Check sheet for the modelled part. Datum: model origin and axes. Units: mm. A direction names the side the tool comes from. Round coordinates to 2 decimals unless told otherwise and drop trailing zeros. Loops run counter-clockwise (first coordinate to the right, second up) from the corner with the lowest first, then second, coordinate; pieces in that order, holes last. Notation, with made-up numbers: (-8, -5) - (23, -5) arc R32 ccw to (23, 26) - close; hole circle Ø3 at (7.25, 71.25). An arc over 180 degrees is marked (long way). Put each result on its own line as item: value. Start each with the question number.
Item 1: Section check C-C, the plane y = 1.25. Give the number of separate pieces and of enclosed holes in the cut face, and give its area (3 significant figures).
Item 2: Tool access check on faces 5 (the flat face through (-23.768, 6, -4)), 6 (the flat face through (-7, 3, 15.211)), 7 (the cylindrical face through (-31.67, 3.11, 14.64)), 8 (the flat face through (3, 2, -2.789)), 9 (the flat face through (7.832, 6, -16)). Record the directions out of +Z, -Z, +X, -X, +Y, -Y that give a thin tool (end or side, any length) a straight path to the whole face; none if there is none.
Item 3: Section check A-A, the plane z = 3.5. Record the cut outline in (x, y), and give its area (3 significant figures).
Item 4: Gauge pin test, flat ends, axial feed: pin 1 Ø0.5 at (x, y) = (0, 2.5) entering from -Z; pin 2 Ø2 at (y, z) = (2.5, -8) entering from -X; pin 3 Ø2 at (y, z) = (3.5, 1) entering from +X; pin 4 Ø3 at (x, y) = (-4.5, 7) entering from -Z. Record the tip position at first contact, or that the pin passes through.
Item 5: Section check B-B, the plane x = 13. Record the cut outline in (y, z), and give its area (3 significant figures).
Item 6: Draft check along Z on faces 1 (the cylindrical face through (17.13, 3.11, 14.64)), 2 (the flat face through (-18, 2, -16.789)), 3 (the flat face through (-32.268, 3, -4)), 4 (the flat face through (-14, 2, -16.789)). Enter one of: pulls with the +Z half, pulls with the -Z half, needs draft (parallel to the pull), parting line crosses it, or undercut.
Item 7: Material ranges on line 1 along Z through (x, y) = (0, 6); line 2 along X through (y, z) = (5, -6.5); line 3 along Y through (x, z) = (2.5, -29), recorded low to high.
from build123d import *
from build123d.topology import SkipClean

# Parameters (mm, degrees)
SKETCH_1_W          = 54
SKETCH_1_H          = 54
EXTRUDE_2_DEPTH     = 2.2
SKETCH_7_W          = 50
SKETCH_7_H          = 50
EXTRUDE_3_DEPTH     = 1.8
EXTRUDE_5_DEPTH     = 4
SKETCH_9_8_W        = 1.5
SKETCH_9_8_H        = 7
SKETCH_9_8_H_2      = 14
CUT_EXTRUDE_2_DEPTH = 10
FILLET_1_R          = 2
SKETCH_15_W         = 0.001
SKETCH_15_H         = 1.8
REVOLVE_8_ANGLE     = 332


with BuildPart() as part:
    # 草图1 → 凸台-拉伸2 (new body)
    with BuildSketch(Plane(origin=(0, 0, 0), x_dir=(1, 0, 0), z_dir=(0, 1, 0))):
        with Locations((-7.2681601, 9.789048154)):
            Rectangle(SKETCH_1_W, SKETCH_1_H)
    extrude(amount=EXTRUDE_2_DEPTH)

    # 草图7 → 凸台-拉伸3 (add)
    with BuildSketch(Plane(origin=(0, 2.2, 0), x_dir=(1, 0, 0), z_dir=(0, 1, 0))):
        with Locations((-7.2681601, 9.789048154)):
            Rectangle(SKETCH_7_W, SKETCH_7_H)
    extrude(amount=EXTRUDE_3_DEPTH)

    # 草图9 → 凸台-拉伸5 (add)
    with BuildSketch(Plane(origin=(0, 4, 0), x_dir=(1, 0, 0), z_dir=(0, 1, 0))):
        with BuildLine():
            Line((-22.7681601, -1.710951846), (8.2318399, -1.710951846))
            ThreePointArc((8.2318399, -1.710951846), (8.938946681, -1.418058627), (9.2318399, -0.710951846))
            Line((9.2318399, -0.710951846), (9.2318399, 7.789048154))
            Line((9.2318399, 7.789048154), (7.8318399, 7.789048154))
            Line((7.8318399, 7.789048154), (7.8318399, -0.310951846))
            Line((7.8318399, -0.310951846), (-22.3681601, -0.310951846))
            Line((-22.3681601, -0.310951846), (-22.3681601, 7.789048154))
            Line((-22.3681601, 7.789048154), (-23.7681601, 7.789048154))
            Line((-23.7681601, 7.789048154), (-23.7681601, -0.710951846))
            ThreePointArc((-23.7681601, -0.710951846), (-23.475266881, -1.418058627), (-22.7681601, -1.710951846))
        make_face()
        with BuildLine():
            Line((-22.7681601, 21.289048154), (8.2318399, 21.289048154))
            ThreePointArc((8.2318399, 21.289048154), (8.938946681, 20.996154935), (9.2318399, 20.289048154))
            Line((9.2318399, 20.289048154), (9.2318399, 11.789048154))
            Line((9.2318399, 11.789048154), (7.8318399, 11.789048154))
            Line((7.8318399, 11.789048154), (7.8318399, 19.889048154))
            Line((7.8318399, 19.889048154), (-22.3681601, 19.889048154))
            Line((-22.3681601, 19.889048154), (-22.3681601, 11.789048154))
            Line((-22.3681601, 11.789048154), (-23.7681601, 11.789048154))
            Line((-23.7681601, 11.789048154), (-23.7681601, 20.289048154))
            ThreePointArc((-23.7681601, 20.289048154), (-23.475266881, 20.996154935), (-22.7681601, 21.289048154))
        make_face()
    extrude(amount=EXTRUDE_5_DEPTH)

    # 草图9<8> → 切除-拉伸2 (cut)
    with BuildSketch(Plane(origin=(0, 4, 0), x_dir=(1, 0, 0), z_dir=(0, 1, 0))):
        with Locations((-10.7681601, 13.289048154)):
            Rectangle(SKETCH_9_8_W, SKETCH_9_8_H)
        with Locations((-10.7681601, 6.289048154)):
            Rectangle(SKETCH_9_8_W, SKETCH_9_8_H)
        with Locations((-7.2681601, 9.789048154)):
            Rectangle(SKETCH_9_8_W, SKETCH_9_8_H_2)
        with Locations((-14.2681601, 9.789048154)):
            Rectangle(SKETCH_9_8_W, SKETCH_9_8_H_2)
        with Locations((-17.7681601, 9.789048154)):
            Rectangle(SKETCH_9_8_W, SKETCH_9_8_H_2)
        with Locations((-3.7681601, 9.789048154)):
            Rectangle(SKETCH_9_8_W, SKETCH_9_8_H_2)
        with Locations((-0.2681601, 9.789048154)):
            Rectangle(SKETCH_9_8_W, SKETCH_9_8_H_2)
        with Locations((3.2318399, 9.789048154)):
            Rectangle(SKETCH_9_8_W, SKETCH_9_8_H_2)
    extrude(amount=-CUT_EXTRUDE_2_DEPTH, mode=Mode.SUBTRACT)

    # 圆角1
    fillet_1_edges = [part.edges().sort_by_distance(p)[0] for p in [
        (17.7318399, 3.1, 15.210951846),
        (17.7318399, 3.1, -34.789048154),
        (-32.2681601, 3.1, -34.789048154),
        (-32.2681601, 3.1, 15.210951846),
        (-34.2681601, 1.1, -36.789048154),
        (19.7318399, 1.1, -36.789048154),
        (19.7318399, 1.1, 17.210951846),
        (-34.2681601, 1.1, 17.210951846),
    ]]
    fillet(fillet_1_edges, radius=FILLET_1_R)

    # 草图12 → 旋转-薄壁5 (revolve)
    with BuildSketch(Plane.XY.offset(15.210951846)):
        with BuildLine():
            ThreePointArc((-7.2681601, 2.35), (-6.5181601, 3.1), (-7.2681601, 3.85))
            Line((-7.2681601, 3.85), (-7.2681601, 3.851))
            ThreePointArc((-7.2681601, 3.851), (-6.5171601, 3.1), (-7.2681601, 2.349))
            Line((-7.2681601, 2.349), (-7.2681601, 2.35))
        make_face()
    revolve(axis=Axis((-7.2681601, 4, 15.210951846), (0, -1, 0)))

    # 草图13 → 旋转-薄壁6 (revolve)
    with BuildSketch(Plane.ZY.offset(32.2681601)):
        with BuildLine():
            ThreePointArc((-9.789048154, 2.35), (-9.039048154, 3.1), (-9.789048154, 3.85))
            Line((-9.789048154, 3.85), (-9.789048154, 3.851))
            ThreePointArc((-9.789048154, 3.851), (-9.038048154, 3.1), (-9.789048154, 2.349))
            Line((-9.789048154, 2.349), (-9.789048154, 2.35))
        make_face()
    revolve(axis=Axis((-32.2681601, 4, -9.789048154), (0, -1, 0)))

    # 草图15 → 旋转-薄壁8 (revolve)
    with SkipClean():  # the faces are left unmerged after this step: merging them gives an invalid solid
        with BuildSketch(Plane(origin=(17.7318399, 0, 0), x_dir=(0, 0, -1), z_dir=(1, 0, 0))):
            with Locations((9.788548154, 3.1)):
                Rectangle(SKETCH_15_W, SKETCH_15_H)
            with BuildLine():
                ThreePointArc((9.789048154, 2.35), (10.539048154, 3.1), (9.789048154, 3.85))
                Line((9.789048154, 3.85), (9.789048154, 3.851))
                ThreePointArc((9.789048154, 3.851), (10.540048154, 3.1), (9.789048154, 2.349))
                Line((9.789048154, 2.349), (9.789048154, 2.35))
            make_face()
        revolve(axis=Axis((17.7318399, 4, -9.789048154), (0, -1, 0)), revolution_arc=REVOLVE_8_ANGLE)
    add(part.part.scale(1), mode=Mode.REPLACE)  # the faces are merged on a copy

    # 草图16 → 旋转-薄壁9 (revolve)
    with BuildSketch(Plane(origin=(0, 0, -34.789048154), x_dir=(-1, 0, 0), z_dir=(0, 0, -1))):
        with BuildLine():
            ThreePointArc((7.2681601, 3.85), (6.5181601, 3.1), (7.2681601, 2.35))
            Line((7.2681601, 2.35), (7.2681601, 2.349))
            ThreePointArc((7.2681601, 2.349), (6.5171601, 3.1), (7.2681601, 3.851))
            Line((7.2681601, 3.851), (7.2681601, 3.85))
        make_face()
    revolve(axis=Axis((-7.2681601, 4, -34.789048154), (0, -1, 0)))


solid = part.part
Check result:
1. separate pieces: 1
1. enclosed holes: 7
1. area: 2,770 mm²
2. face 5: +Z, -Z, -X, +Y
2. face 6: none
2. face 7: +Z, -X, +Y
2. face 8: +Y, -Y
2. face 9: +Y
3. outline: (-34.27, 0) - (19.73, 0) - (19.73, 2.2) - (17.73, 2.2) - (17.73, 4) - (-32.27, 4) - (-32.27, 2.2) - (-34.27, 2.2) - close
3. area: 209 mm²
4. pin 1: z = -34.79
4. pin 2: x = -34.27
4. pin 3: x = 17.73
4. pin 4: z = -21.29
5. outline: (0, -36.79) - (2.2, -36.79) - (2.2, -34.79) - (4, -34.79) - (4, 15.21) - (2.2, 15.21) - (2.2, 17.21) - (0, 17.21) - close
5. area: 209 mm²
6. face 1: pulls with the +Z half
6. face 2: undercut
6. face 3: needs draft
6. face 4: undercut
7. line 1: -21.29 to -19.89, 0.31 to 1.71
7. line 2: -23.77 to -22.37, 7.83 to 9.23
7. line 3: 0 to 4
